Design review of the part shown in the three views and the two pictorial views. Dimensions are in mm from the part's minimum x, y and z. Round coordinates to 2 decimals unless told otherwise and drop trailing zeros. Order: outer loops, then holes, each group sorted by start corner. A loop starts at its lowest first (then second) coordinate and runs counter-clockwise, first axis right, second up.
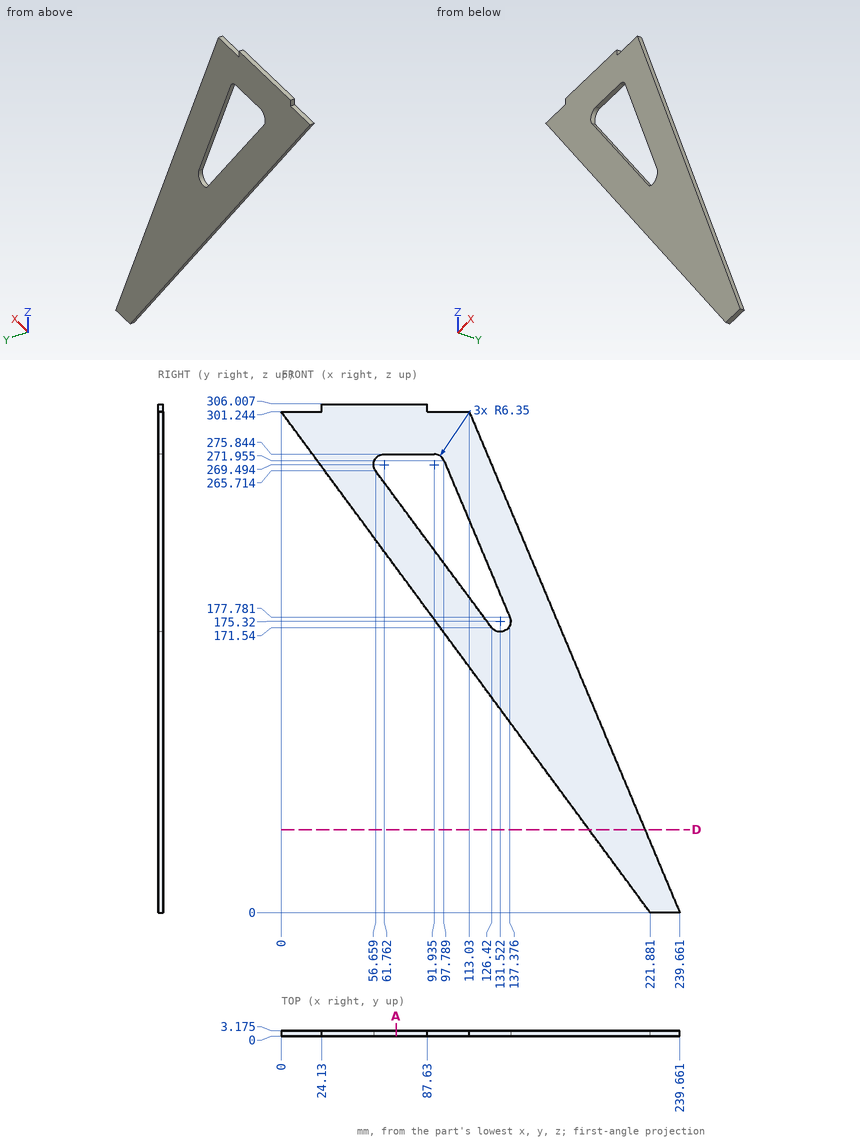
(1) Wall thickness on L1, parallel to Z at x = 60.5, y = 2.1 (1 decimal); L2, parallel to X at y = 1.05, z = 169.5 (1 decimal); L3, parallel to X at y = 1.8, z = 224.5 (1 decimal): over which ranges is each line inside the solid? List them lowest first.
(2) Add section A-A on x = 69. Give the boundary of the cut face in (y, z) (1 decimal).
(3) Add section D-D on z = 50. Give the boundary of the cut face in (x, y) (1 decimal), plus the area to 3 significant figures.
(4) Clearance check with flat-ended pins moving along their axes: P1, Ø1.5, axis at y = 2.5, z = 79.5, coming from the -X side; P2, Ø1.6, axis at x = 70.5, y = 2, coming from the -Z side; P3, Ø1, axis at x = 158, y = 2, coming from the -Z side. State where each tip first meets the part, or that it passes through.
Here are the results:
1. L1: z = 219.1 to 260.5, 275.7 to 306
1. L2: x = 97 to 129, 134.1 to 168.4
1. L3: x = 56.5 to 87.2, 117.7 to 145.3
2. outline: (0, 207.6) - (3.2, 207.6) - (3.2, 249.1) - (0, 249.1) - close; (0, 275.8) - (3.2, 275.8) - (3.2, 306) - (0, 306) - close
3. outline: (185.1, 0) - (218.6, 0) - (218.6, 3.2) - (185.1, 3.2) - close
3. area: 107 mm2
4. P1: stops at x = 162.77
4. P2: stops at z = 204.44
4. P3: stops at z = 86.05
